from build123d import *

# Parameters (mm, degrees)
F0_W     = 40
F0_H     = 12
F1_DEPTH = 50
F3_DEPTH = 55
F4_R     = 6.5
F5_DEPTH = 13
F6_SIZE  = 0.8


# Not quite as in the source:
# - a feature names something its author has since deleted; it is built from what else it names


with BuildPart() as f1:
    # F0 (on Top) → F1 (new body)
    with BuildSketch(Plane.XY):
        with Locations((-12.258, 6)):
            Rectangle(F0_W, F0_H)
    extrude(amount=F1_DEPTH)

    # F2 (on face) → F3 (cut)
    with BuildSketch(Plane.XY.offset(50)):
        with BuildLine():
            Line((-25.258, 9), (-27.258, 9))
            ThreePointArc((-27.258, 9), (-30.258, 6), (-27.258, 3))
            Line((-27.258, 3), (-25.258, 3))
            ThreePointArc((-25.258, 3), (-22.258, 6), (-25.258, 9))
        make_face()
        with BuildLine():
            Line((0.742, 3), (2.742, 3))
            ThreePointArc((2.742, 3), (5.742, 6), (2.742, 9))
            Line((2.742, 9), (0.742, 9))
            ThreePointArc((0.742, 9), (-2.258, 6), (0.742, 3))
        make_face()
    extrude(amount=-F3_DEPTH, mode=Mode.SUBTRACT)

    # F4 (on face) → F5 (cut)
    with BuildSketch(Plane.XZ):
        with Locations((-13.208, 25)):
            Circle(F4_R)
    extrude(amount=-F5_DEPTH, mode=Mode.SUBTRACT)

    # F6
    f6_edges = [f1.edges().sort_by_distance(p)[0] for p in [
        (7.742, 0, 25),
        (-32.258, 12, 25),
        (-32.258, 0, 25),
        (-19.708, 12, 25),
        (-19.708, 0, 25),
        (7.742, 12, 25),
    ]]
    chamfer(f6_edges, length=F6_SIZE)


solid = f1.part
Model file for the job. Use its own axes, mm. A direction names the side the tool comes from. Round coordinates to 2 decimals unless told otherwise and drop trailing zeros. Order: outer loops, then holes, each group sorted by start corner. A loop starts at its lowest first (then second) coordinate and runs counter-clockwise, first axis right, second up.
(1) Band-saw the part on D-D (x = -26.5). List the corners of the cut face in (y, z).
(2) Band-saw the part on A-A (y = 6). List the corners of the cut face in (x, z).
(3) Band-saw the part on B-B (z = 25). List the corners of the cut face in (x, y), then the cut area to 3 significant figures.
(4) Band-saw the part on C-C (z = 4.5). List the corners of the cut face in (x, y).
(5) Drill centre lines: line 1 (Y direction, x = -26, z = 20); line 2 (X direction, y = 3.5, z = 26); line 3 (X direction, y = 6.75, z = 19). Where is each one in solid material? Low to high.
(6) Pull direction Y, two halves, no side cores. Call faces 3 (the face through (5.74, 5.93, 25.35)), 4 (the face through (-8, 0, 19)), 5 (the face through (-13, 6, 50)), 6 (the face through (-8, 12, 19)): released by +Y, released by -Y, zero draft, split by the parting line, or undercut.
(7) 3-axis set-ups, long thin cutter, end or side, ignore diameter. For faces 1 (the face through (-26, 9, 25)), 2 (the face through (-7.008, 5.927, 26.952)): which of +Z, -Z, +X, -X, +Y, -Y reach the whole face in a straight line?
Verdict:
1. outline: (0, 0) - (3, 0) - (3, 50) - (0, 50) - close; (9, 0) - (12, 0) - (12, 50) - (9, 50) - close
2. outline: (-32.26, 0) - (-30.26, 0) - (-30.26, 50) - (-32.26, 50) - close; (-22.26, 0) - (-2.26, 0) - (-2.26, 50) - (-22.26, 50) - close; (5.74, 0) - (7.74, 0) - (7.74, 50) - (5.74, 50) - close; hole circle Ø13 at (-13.21, 25)
3. outline: (-32.26, 0.8) - (-31.46, 0) - (-20.51, 0) - (-19.71, 0.8) - (-19.71, 11.2) - (-20.51, 12) - (-31.46, 12) - (-32.26, 11.2) - close; (-6.71, 0.8) - (-5.91, 0) - (6.94, 0) - (7.74, 0.8) - (7.74, 11.2) - (6.94, 12) - (-5.91, 12) - (-6.71, 11.2) - close; hole (-27.26, 3) - (-25.26, 3) arc R3 ccw to (-25.26, 9) - (-27.26, 9) arc R3 ccw to start; hole (0.74, 3) - (2.74, 3) arc R3 ccw to (2.74, 9) - (0.74, 9) arc R3 ccw to start
3. area: 241 mm2
4. outline: (-32.26, 0.8) - (-31.46, 0) - (6.94, 0) - (7.74, 0.8) - (7.74, 11.2) - (6.94, 12) - (-31.46, 12) - (-32.26, 11.2) - close; hole (-27.26, 3) - (-25.26, 3) arc R3 ccw to (-25.26, 9) - (-27.26, 9) arc R3 ccw to start; hole (0.74, 3) - (2.74, 3) arc R3 ccw to (2.74, 9) - (0.74, 9) arc R3 ccw to start
5. line 1: y = 0 to 3, 9 to 12
5. line 2: x = -32.26 to -28.92, -23.6 to -19.63, -6.79 to -0.92, 4.4 to 7.74
5. line 3: x = -32.26 to -30.16, -22.35 to -15.71, -10.71 to -2.16, 5.65 to 7.74
6. face 3: undercut
6. face 4: released by -Y
6. face 5: zero draft
6. face 6: released by +Y
7. face 1: +Z, -Z
7. face 2: +Y, -Y
